Input: part model. Units: mm. Frame: model coordinates. A direction names the side the tool comes from. Give positions to 0.01 mm unless a question says otherwise; leave off trailing zeros. Loops run counter-clockwise (first coordinate to the right, second up) from the corner with the lowest first, then second, coordinate; pieces in that order, holes last. Notation, with made-up numbers: M -25,46.25 L 15,46.25 A26 cw 15,69.25 Z; hole C -19.5,-31.75 d7. An arc over 180 degrees is marked long. Answer as a JSON object with one key per item and string values. Group by question number.
1) First-contact query: P1, Ø4, axis at y = -1.5, z = -6.5, coming from the -X side; P2, Ø2.5, axis at x = 0, y = -0.5, coming from the -Z side; P3, Ø1.5, axis at x = 2, z = -1, coming from the +Y side. Flat tips, straight axial feed; report the tip coordinate or a pass-through.
2) Section query B-B on x = -0.5. Return loops of the section in (y, z).
3) Section query D-D on x = -3.5. Return loops of the section in (y, z), plus the area to 3 significant figures.
4) Section query A-A on y = 0. Return loops of the section in (x, z) (3 decimals), plus the area to 3 significant figures.
5) Ray query, L1, parallel to X at y = 0, z = -5.65; L2, parallel to Z at x = -3.75, y = 0.25; L3, parallel to Y at x = -0.5, z = -5.75. Return the intervals inside material, ascending.
6) Section query C-C on z = 3.25. Return loops of the section in (x, y) (3 decimals).
7) Draft query along X for faces 1 (the cylindrical face through (-2.44, -0.54, -6.52)), 2 (the cylindrical face through (-3.905, -0.867, -4.451)), 3 (the flat face through (-2.2, -2.2, 0)). Return one class per face: +X half, -X half, draft (parallel to the pull), parting line (faces both ways), or undercut.
8) Access query for faces 4 (the flat face through (2, 2, -8)), 5 (the flat face through (0, 0, -5)), 6 (the cylindrical face through (-0.37, 2.85, 2.96)). Directions: +Z, -Z, +X, -X, +Y, -Y. A direction counts if a zero-diameter tool reaches every point of the face in a straight line with its end or side. Return the directions, or none.
from build123d import *

# Parameters (mm, degrees)
SKETCH13_R          = 5
BOSS_EXTRUDE5_DEPTH = 1
SKETCH14_R          = 4
BOSS_EXTRUDE6_DEPTH = 7
SKETCH15_R          = 2.5
CUT_EXTRUDE5_DEPTH  = 3
SKETCH16_R          = 2.875
BOSS_EXTRUDE7_DEPTH = 6


with BuildPart() as part:
    # Sketch13 → Boss-Extrude5 (new body)
    with BuildSketch(Plane(origin=(0, 5, 0), x_dir=(1, 0, 0), z_dir=(0, 0, -1))):
        with Locations(Location((0, 5, 0), (0, 0, 180))):
            Circle(SKETCH13_R)
    extrude(amount=BOSS_EXTRUDE5_DEPTH)

    # Sketch14 → Boss-Extrude6 (add)
    with BuildSketch(Plane(origin=(0, 0, -1), x_dir=(1, 0, 0), z_dir=(0, 0, -1))):
        with Locations(Location((0, 0, 0), (0, 0, 270))):
            Circle(SKETCH14_R)
    extrude(amount=BOSS_EXTRUDE6_DEPTH)

    # Sketch15 → Cut-Extrude5 (cut)
    with BuildSketch(Plane(origin=(0, 0, -8), x_dir=(1, 0, 0), z_dir=(0, 0, -1))):
        with Locations(Location((0, 0, 0), (0, 0, 270))):
            Circle(SKETCH15_R)
    extrude(amount=-CUT_EXTRUDE5_DEPTH, mode=Mode.SUBTRACT)

    # Sketch16 → Boss-Extrude7 (add)
    with BuildSketch(Plane.XY):
        Circle(SKETCH16_R)
    extrude(amount=BOSS_EXTRUDE7_DEPTH)


solid = part.part
Output:
{
 "1": {"P1": "stops at x = -4", "P2": "stops at z = -5", "P3": "stops at y = 4.84"},
 "2": {"outline": "M -4.97,-1 L -3.97,-1 L -3.97,-8 L -2.45,-8 L -2.45,-5 L 2.45,-5 L 2.45,-8 L 3.97,-8 L 3.97,-1 L 4.97,-1 L 4.97,0 L 2.83,0 L 2.83,6 L -2.83,6 L -2.83,0 L -4.97,0 Z"},
 "3": {"outline": "M -3.57,-1 L -1.94,-1 L -1.94,-8 L 1.94,-8 L 1.94,-1 L 3.57,-1 L 3.57,0 L -3.57,0 Z", "area": "34.3 mm^2"},
 "4": {"outline": "M -5,-1 L -4,-1 L -4,-8 L -2.5,-8 L -2.5,-5 L 2.5,-5 L 2.5,-8 L 4,-8 L 4,-1 L 5,-1 L 5,0 L 2.875,0 L 2.875,6 L -2.875,6 L -2.875,0 L -5,0 Z", "area": "85.5 mm^2"},
 "5": {"L1": "x = -4 to -2.5, 2.5 to 4", "L2": "z = -8 to 0", "L3": "y = -3.97 to -2.45, 2.45 to 3.97"},
 "6": {"outline": "C 0,0 d5.75"},
 "7": {"face 1": "undercut", "face 2": "parting line", "face 3": "draft"},
 "8": {"face 4": "-Z, +X, -X, +Y, -Y", "face 5": "-Z", "face 6": "+Z"}
}
